from build123d import *

# Parameters (mm, degrees)
EXTRUDE_1_DEPTH          = 7.5
CUT_EXTRUDE_3_DEPTH      = 8.5
CUT_EXTRUDE_3_DEPTH_BACK = 8.5
HOLE_WIZARD_M4_1_D       = 6.6


with BuildPart() as part:
    # 스케치1 → 보스-돌출1 (new body, symmetric)
    with BuildSketch(Plane.XY):
        Polygon((-14, 22), (14, 22), (14, 6), (40, 6), (40, 0), (-40, 0), (-40, 6), (-14, 6), align=None)
    extrude(amount=EXTRUDE_1_DEPTH, both=True)

    # 스케치2 → 컷-돌출3 (cut, two sides)
    with BuildSketch(Plane.XY) as cut_extrude_3_sk:
        with BuildLine():
            Line((-40, 0), (-31.112698372, 0))
            ThreePointArc((-31.112698372, 0), (0, 22), (31.112698372, 0))
            Line((31.112698372, 0), (40, 0))
            Line((40, 0), (40, 32))
            Line((40, 32), (-40, 32))
            Line((-40, 32), (-40, 0))
        make_face()
    extrude(amount=CUT_EXTRUDE_3_DEPTH, mode=Mode.SUBTRACT)
    extrude(cut_extrude_3_sk.sketch, amount=-CUT_EXTRUDE_3_DEPTH_BACK, mode=Mode.SUBTRACT)

    # M4 여유 구멍1 (through all)
    with Locations(Plane(origin=(0, 6, 0), x_dir=(1, 0, 0), z_dir=(0, 1, 0))):
        with Locations((-21, 0), (21, 0)):
            Hole(HOLE_WIZARD_M4_1_D / 2)


solid = part.part
Build history of the part. All positions in model axes, mm. A direction names the side the tool comes from. Coordinates: 2 decimals unless noted, no trailing zeros. Order: outer loops, then holes, each group sorted by start corner. A loop starts at its lowest first (then second) coordinate and runs counter-clockwise, first axis right, second up. Notation, with made-up numbers: (11.5, 22.25) - (42.5, 22.25) arc R28 cw to (42.5, 61.25) - close; hole circle Ø7 at (79, 74.5). An arc over 180 degrees is marked (long way). Write item = value, one per line. Start each with the question number.
1) Saw through at A-A on z = 0. Write the cut outline in (x, y).
2) Saw through at D-D on x = -6. Write the cut outline in (y, z).
3) Flat gauge pins, fed straight in: pin 1 Ø4.5 at (x, z) = (19, 3.5) entering from +Y; pin 2 Ø4 at (x, z) = (-11.5, 3) entering from +Y; pin 3 Ø4 at (y, z) = (11.5, -1.5) entering from +X. Where does each tip first touch, or does it go through?
4) Two-plate mould, pull along Z, no slides. Class faces 4 (the face through (-14, 12, 0)), 5 (the face through (-24.05, 2.96, 1.26)), 6 (the face through (0, 9, -7.5)): pulls with the +Z half, pulls with the -Z half, needs draft (parallel to the pull), parting line crosses it, or undercut.
5) Saw through at B-B on x = 21. Write the cut outline in (y, z).
6) Wall check: line 1 along Z through (x, y) = (-21, 4); line 2 along X through (y, z) = (15.25, 6); line 3 along X through (y, z) = (4, 2.5). Give the ranges that are in metal, low to high. Write a range as from..to.
7) Saw through at C-C on y = 10.5. Write the cut outline in (x, z), then the cut area to 3 significant figures.
8) 3-axis set-ups, long thin cutter, end or side, ignore diameter. For faces 1 (the face through (24, 6, 2)), 2 (the face through (0, 22, 0)), 3 (the face through (-24, 6, 2)): which of +Z, -Z, +X, -X, +Y, -Y reach the whole face in a straight line?
From the geometry:
q1.outline = (-31.11, 0) - (-24.3, 0) - (-24.3, 6) - (-28.28, 6) arc R33 ccw to start; (-17.7, 0) - (17.7, 0) - (17.7, 6) - (14, 6) - (14, 18.88) arc R33 ccw to (-14, 18.88) - (-14, 6) - (-17.7, 6) - close; (24.3, 0) - (31.11, 0) arc R33 ccw to (28.28, 6) - (24.3, 6) - close
q2.outline = (0, -7.5) - (21.45, -7.5) - (21.45, 7.5) - (0, 7.5) - close
q3.pin_1 = 6
q3.pin_2 = 20.6
q3.pin_3 = 14
q4.face_4 = needs draft
q4.face_5 = undercut
q4.face_6 = pulls with the -Z half
q5.outline = (0, -7.5) - (6, -7.5) - (6, -3.3) - (0, -3.3) - close; (0, 3.3) - (6, 3.3) - (6, 7.5) - (0, 7.5) - close
q6.line_1 = -7.5..-3.3, 3.3..7.5
q6.line_2 = -14..14
q6.line_3 = -29.39..-23.15, -18.85..18.85, 23.15..29.39
q7.outline = (-14, -7.5) - (14, -7.5) - (14, 7.5) - (-14, 7.5) - close
q7.area = 420 mm^2
q8.face_1 = +Z, -Z, +X, +Y
q8.face_2 = +Z, -Z, +Y
q8.face_3 = +Z, -Z, -X, +Y
